Input: part model. Units: mm. Frame: model coordinates. A direction names the side the tool comes from. Give positions to 0.01 mm unless a question says otherwise; leave off trailing zeros. Write each loop counter-clockwise with the first axis right and the second up, starting at its lowest first coordinate (ties: lowest second). Pieces come first, ordered by that corner, then holes.
```python
from build123d import *

# Parameters (mm, degrees)
SZKIC1_W                                          = 22
SZKIC1_H                                          = 20
DODANIE_WYCI_GNI_CIE1_DEPTH                       = 8
WYTNIJ_WYCI_GNI_CIE1_DEPTH                        = 8
WYTNIJ_WYCI_GNI_CIE2_DEPTH                        = 31.789608637
WYTNIJ_WYCI_GNI_CIE2_DEPTH_BACK                   = 31.789608637
POG_BIENIE_WALCOWE_POD_M5_RUB_Z_BEM_W_D           = 5.5
POG_BIENIE_WALCOWE_POD_M5_RUB_Z_BEM_W_CBORE_D     = 10
POG_BIENIE_WALCOWE_POD_M5_RUB_Z_BEM_W_CBORE_DEPTH = 5
ZAOKR_GLENIE1_R                                   = 3
ZAOKR_GLENIE2_R                                   = 1


with BuildPart() as part:
    # Szkic1 → Dodanie-wyciągnięcie1 (new, symmetric)
    with BuildSketch(Plane.XY):
        with Locations((11, 10)):
            Rectangle(SZKIC1_W, SZKIC1_H)
    dodanie_wyci_gni_cie1 = extrude(amount=DODANIE_WYCI_GNI_CIE1_DEPTH, both=True)

    # Lustro1: Dodanie-wyciągnięcie1 across plane
    add(dodanie_wyci_gni_cie1.mirror(Plane(origin=(0, 20, 8), x_dir=(0, 0, 1), z_dir=(1, 0, 0))))

    # Szkic2 → Wytnij-wyciągnięcie1 (cut)
    with BuildSketch(Plane.XY.offset(8)):
        with BuildLine():
            Line((-13, 20), (13, 20))
            ThreePointArc((13, 20), (0, 7), (-13, 20))
        make_face()
    extrude(amount=-WYTNIJ_WYCI_GNI_CIE1_DEPTH, mode=Mode.SUBTRACT)

    # Szkic3 → Wytnij-wyciągnięcie2 (cut, two sides: drawn at the far end of the back side and taken through both)
    with BuildSketch(Plane.XY.offset(-WYTNIJ_WYCI_GNI_CIE2_DEPTH_BACK)):
        with BuildLine():
            ThreePointArc((-9, 20), (0, 11), (9, 20))
            Line((9, 20), (-9, 20))
        make_face()
    extrude(amount=WYTNIJ_WYCI_GNI_CIE2_DEPTH + WYTNIJ_WYCI_GNI_CIE2_DEPTH_BACK, mode=Mode.SUBTRACT)

    # Pogłębienie walcowe pod M5 Śrubę z łbem walcowym z gniazdem1 (through all)
    with Locations(Plane(origin=(0, 0, 0), x_dir=(-1, 0, 0), z_dir=(0, -1, 0))):
        with Locations((-17.5, 0), (17.5, 0)):
            CounterBoreHole(POG_BIENIE_WALCOWE_POD_M5_RUB_Z_BEM_W_D / 2, POG_BIENIE_WALCOWE_POD_M5_RUB_Z_BEM_W_CBORE_D / 2, POG_BIENIE_WALCOWE_POD_M5_RUB_Z_BEM_W_CBORE_DEPTH)

    # Zaokrąglenie1
    zaokr_glenie1_edges = [part.edges().sort_by_distance(p)[0] for p in [
        (-22, 0, 5.089724736),
        (-22, 0, -5.089724736),
        (22, 0, -5.089724736),
        (22, 0, 5.089724736),
    ]]
    fillet(zaokr_glenie1_edges, radius=ZAOKR_GLENIE1_R)

    # Zaokrąglenie2
    zaokr_glenie2_edges = [part.edges().sort_by_distance(p)[0] for p in [
        (-22, 11.5, 8),
        (-21.121320344, 0.878679656, 8),
        (0, 0, 8),
        (21.121320344, 0.878679656, 8),
        (0, 0, -8),
        (0, 11, -8),
        (22, 11.5, 8),
        (0, 11, 0),
        (22, 11.5, -8),
        (-21.121320344, 0.878679656, -8),
        (21.121320344, 0.878679656, -8),
    ]]
    fillet(zaokr_glenie2_edges, radius=ZAOKR_GLENIE2_R)


solid = part.part
```
Q1. Section C-C, the plane z = 1. Return the cut outline in (x, y), then the cut area to 3 significant figures.
Q2. Section B-B, the plane y = 6.25. Return the cut outline in (x, z).
Q3. Pin query (flat end, axial travel): pin 1 (7 mm diameter, centred on x = -17.5, z = 0, fed in from -Y); pin 2 (4 mm diameter, centred on x = -3.5, y = 11.5, fed in from +Z). Return the tip coordinate at first contact, or that it passes through.
Q4. Section A-A, the plane x = -17.5. Return the cut outline in (y, z).
Q5. Section D-D, the plane x = 0. Return the cut outline in (y, z), then the cut area to 3 significant figures.
Q6. Mould query, pull axis Z, two halves, no side actions, for faces 4 (the cylindrical face through (-21.699, 11.619, 7.715)), 5 (the cylindrical face through (-12.504, 2.465, -0.188)), 6 (the flat face through (22, 11, 0)). Classes: +Z half, -Z half, draft (parallel to the pull), parting line (faces both ways), or undercut.
Q7. Access query for faces 1 (the flat face through (0.1, 9.7, 0)), 2 (the cylindrical face through (-21.48, 1.31, 5.16)), 3 (the flat face through (-19.3, 5, -2.3)). Directions: +Z, -Z, +X, -X, +Y, -Y. A direction counts if a zero-diameter tool reaches every point of the face in a straight line with its end or side. Return the directions, or none.
Q8. Material intervals for line 1 along Z through (x, y) = (17.5, 15.25); line 2 along Z through (x, y) = (17.5, 3.6); line 3 along X through (y, z) = (8, 4.25), sorted ascending.
Solutions:
1. outline: (-22, 5) - (-20.06, 5) - (-20.06, 20) - (-22, 20) - close; (-14.94, 5) - (-12.6, 5) - (-12.6, 0) - (12.6, 0) - (12.6, 5) - (14.94, 5) - (14.94, 20) - (13, 20) arc R13 cw to (-13, 20) - (-14.94, 20) - close; (20.06, 5) - (22, 5) - (22, 20) - (20.06, 20) - close
1. area: 367 mm2
2. outline: (-22, -7) arc R1 ccw to (-21, -8) - (21, -8) arc R1 ccw to (22, -7) - (22, 7) arc R1 ccw to (21, 8) - (-21, 8) arc R1 ccw to (-22, 7) - close; hole circle Ø5.5 at (-17.5, 0); hole circle Ø5.5 at (17.5, 0)
3. pin 1: stops at y = 5
3. pin 2: stops at z = 0
4. outline: (0, -7) arc R1 ccw to (1, -8) - (20, -8) - (20, -2.75) - (5, -2.75) - (5, -5) - (0, -5) - close; (0, 5) - (5, 5) - (5, 2.75) - (20, 2.75) - (20, 8) - (1, 8) arc R1 ccw to (0, 7) - close
5. outline: (0, -7) arc R1 ccw to (1, -8) - (10, -8) arc R1 ccw to (11, -7) - (11, -1) arc R1 ccw to (10, 0) - (7, 0) - (7, 8) - (1, 8) arc R1 ccw to (0, 7) - close
5. area: 143 mm2
6. face 4: +Z half
6. face 5: undercut
6. face 6: draft
7. face 1: +Z, +Y
7. face 2: +Z, -Z, -X, -Y
7. face 3: -Y
8. line 1: z = -8 to -2.75, 2.75 to 8
8. line 2: z = -8 to -5, 5 to 8
8. line 3: x = -22 to -5, 5 to 22
